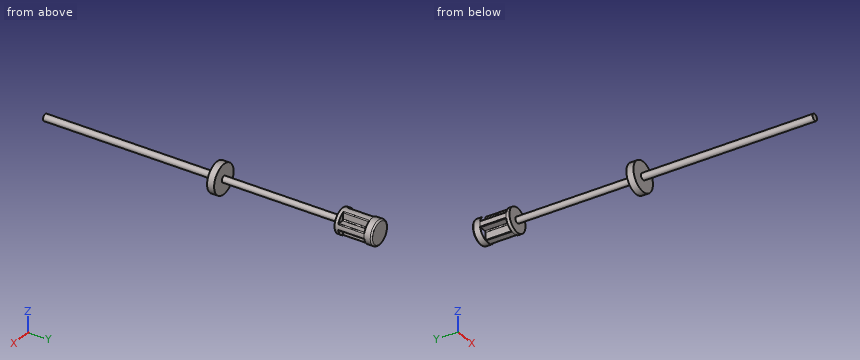
from build123d import *

# Parameters (mm, degrees)
SKETCH1_R           = 0.95
SKETCH5_W           = 4.2
SKETCH5_H           = 2
SKETCH6_R           = 0.885
BOSS_EXTRUDE1_DEPTH = 33.75
SKETCH7_R           = 3.45
BOSS_EXTRUDE2_DEPTH = 1
BOSS_EXTRUDE3_DEPTH = 7.4
SKETCH11_R          = 3.45
BOSS_EXTRUDE4_DEPTH = 2.15
SKETCH12_R          = 5.053108697
SKETCH12_R_2        = 3.449578042
CUT_EXTRUDE1_DEPTH  = 10
FILLET4_R           = 0.4
FILLET5_R           = 0.3
CUT_EXTRUDE2_START  = -3.09
SKETCH15_R          = 0.95
CUT_EXTRUDE2_DEPTH  = 3.09


with BuildPart() as part:
    # Sweep1: sweep along a path in Sketch2
    with BuildLine(Plane(origin=(0, 0, 0), x_dir=(0, 0, -1), z_dir=(1, 0, 0))) as sweep1_path:
        Line((0, 0), (0, 41.9))
        Line((0, 41.9), (0, 51.9))
    # Sketch1 → Sweep1 (sweep)
    with BuildSketch(Plane(origin=(0, 0, 0), x_dir=(1, 0, 0), z_dir=(0, 1, 0))):
        Circle(SKETCH1_R)
    sweep(path=sweep1_path.line)

    # Sketch5 → Revolve1 (revolve)
    with BuildSketch(Plane(origin=(0, 0, 0), x_dir=(0, 0, -1), z_dir=(1, 0, 0))):
        with Locations((-2.1, 52.9)):
            Rectangle(SKETCH5_W, SKETCH5_H)
    revolve(axis=Axis((0, 53.9, 0), (0, -1, 0)))

    # Sketch6 → Boss-Extrude1 (add)
    with BuildSketch(Plane(origin=(0, 53.9, 0), x_dir=(1, 0, 0), z_dir=(0, 1, 0))):
        with Locations(Location((0, 0, 0), (0, 0, 270))):
            Circle(SKETCH6_R)
    extrude(amount=BOSS_EXTRUDE1_DEPTH)

    # Sketch7 → Boss-Extrude2 (add)
    with BuildSketch(Plane(origin=(0, 87.65, 0), x_dir=(1, 0, 0), z_dir=(0, 1, 0))):
        with Locations(Location((0, 0, 0), (0, 0, 270))):
            Circle(SKETCH7_R)
    extrude(amount=BOSS_EXTRUDE2_DEPTH)

    # Sketch8 → Boss-Extrude3 (add)
    with BuildSketch(Plane(origin=(0, 88.65, 0), x_dir=(1, 0, 0), z_dir=(0, 1, 0))):
        Polygon((1.230053166, 0.811701691), (1.230053166, 3.298725541), (-1.010400815, 3.298725541), (-1.010400815, 0.811701691), (-3.353153794, 0.811701691), (-3.353153794, -0.988158581), (-1.010400815, -0.988158581), (-1.010400815, -4.015839789), (1.230053166, -4.015839789), (1.230053166, -0.988158581), (4.082100271, -0.988158581), (4.082100271, 0.811701691), align=None)
    extrude(amount=BOSS_EXTRUDE3_DEPTH)

    # Sketch11 → Boss-Extrude4 (add)
    with BuildSketch(Plane(origin=(0, 96.05, 0), x_dir=(1, 0, 0), z_dir=(0, 1, 0))):
        with Locations(Location((0, 0, 0), (0, 0, 107.029845203))):
            Circle(SKETCH11_R)
    extrude(amount=BOSS_EXTRUDE4_DEPTH)

    # Sketch12 → Cut-Extrude1 (cut)
    with BuildSketch(Plane(origin=(0, 96.05, 0), x_dir=(1, 0, 0), z_dir=(0, 1, 0))):
        Circle(SKETCH12_R)
        with Locations(Location((0, 0, 0), (0, 0, 270))):
            Circle(SKETCH12_R_2, mode=Mode.SUBTRACT)
    extrude(amount=-CUT_EXTRUDE1_DEPTH, mode=Mode.SUBTRACT)

    # Fillet4
    fillet4_edges = [part.edges().sort_by_distance(p)[0] for p in [
        (1.010400815, 98.2, 3.298725541),
    ]]
    fillet(fillet4_edges, radius=FILLET4_R)

    # Fillet5
    # the kernel refuses this fillet: 0.3 mm, written as the material it adds along each edge
    with BuildSketch(Plane(origin=(-1.010400815, 87.9, -0.811701691), x_dir=(-1, 0, 0), z_dir=(0, 1, 0)), Plane(origin=(-1.010400815, 87.9, 0.988158581), x_dir=(0, 0, 1), z_dir=(0, 1, 0)), Plane(origin=(1.230053166, 87.9, -0.811701691), x_dir=(0, 0, -1), z_dir=(0, 1, 0)), Plane(origin=(1.230053166, 87.9, 0.988158581), x_dir=(1, 0, 0), z_dir=(0, 1, 0))) as fillet5_piece_1:
        with BuildLine():
            CenterArc((FILLET5_R, -FILLET5_R), FILLET5_R, 90, 90)
            Line((0, -FILLET5_R), (0, 0))
            Line((0, 0), (FILLET5_R, 0))
        make_face()
    extrude(amount=8.9)
    # the kernel refuses this fillet: 0.3 mm, written as the material it takes off along each edge
    with BuildSketch(Plane(origin=(1.230053166, 88.65, -3.222818313), x_dir=(-0.9453321678939596, 0, -0.32610901911003093), z_dir=(0, 1, 0))) as fillet5_2_piece_1:
        with BuildLine():
            CenterArc((0.213912859, 0.299842347), FILLET5_R, 199.032778114, 72.824800523)
            Line((-0.069686792, 0.202009641), (0, 0))
            ThreePointArc((0, 0), (0.111818707, -0.001812788), (0.223637414, 0))
        make_face()
    extrude(amount=7.4, mode=Mode.SUBTRACT)
    with BuildSketch(Plane(origin=(-1.010400815, 88.65, -3.29828423), x_dir=(0.9657732786653868, 0, -0.2593876909491066), z_dir=(0, 1, 0))) as fillet5_2_piece_2:
        with BuildLine():
            CenterArc((0.230106816, -0.299817566), FILLET5_R, 88.00174108, 76.964525917)
            Line((-0.059625168, -0.222001259), (0, 0))
            ThreePointArc((0, 0), (0.120283777, 0.002097733), (0.240567554, 0))
        make_face()
    extrude(amount=7.4, mode=Mode.SUBTRACT)
    with BuildSketch(Plane(origin=(-3.352719647, 88.65, -0.811701691), x_dir=(-0.1990231654762503, 0, 0.9799947854982765), z_dir=(0, 1, 0))) as fillet5_2_piece_3:
        with BuildLine():
            CenterArc((0.24524038, 0.299792772), FILLET5_R, 191.479842228, 80.649895998)
            Line((-0.048758056, 0.240085822), (0, 0))
            ThreePointArc((0, 0), (0.128194548, -0.002382831), (0.256389095, 0))
        make_face()
    extrude(amount=7.4, mode=Mode.SUBTRACT)
    with BuildSketch(Plane(origin=(-3.30501608, 88.65, 0.988158581), x_dir=(-0.2526309264333675, 0, -0.9675627189022004), z_dir=(0, 1, 0))) as fillet5_2_piece_4:
        with BuildLine():
            CenterArc((0.231775654, -0.29981491), FILLET5_R, 87.987242866, 77.37950549)
            Line((-0.058493162, -0.224025632), (0, 0))
            ThreePointArc((0, 0), (0.121156129, 0.00212828), (0.242312258, 0))
        make_face()
    extrude(amount=7.4, mode=Mode.SUBTRACT)
    with BuildSketch(Plane(origin=(-1.010400815, 88.65, 3.29828423), x_dir=(0.9657732786653864, 0, 0.25938769094910785), z_dir=(0, 1, 0))) as fillet5_2_piece_5:
        with BuildLine():
            CenterArc((0.230106816, 0.299817566), FILLET5_R, 195.033733003, 76.964525917)
            Line((-0.059625168, 0.222001259), (0, 0))
            ThreePointArc((0, 0), (0.120283777, -0.002097733), (0.240567554, 0))
        make_face()
    extrude(amount=7.4, mode=Mode.SUBTRACT)
    with BuildSketch(Plane(origin=(1.230053166, 88.65, 3.222818313), x_dir=(-0.9453321678939602, 0, 0.32610901911002915), z_dir=(0, 1, 0))) as fillet5_2_piece_6:
        with BuildLine():
            CenterArc((0.213912859, -0.299842347), FILLET5_R, 88.142421362, 72.824800523)
            Line((-0.069686792, -0.202009641), (0, 0))
            ThreePointArc((0, 0), (0.111818707, 0.001812788), (0.223637414, 0))
        make_face()
    extrude(amount=7.4, mode=Mode.SUBTRACT)
    with BuildSketch(Plane(origin=(3.30501608, 88.65, 0.988158581), x_dir=(0.2526309264333699, 0, -0.9675627189021997), z_dir=(0, 1, 0))) as fillet5_2_piece_7:
        with BuildLine():
            CenterArc((0.231775654, 0.29981491), FILLET5_R, 194.633251644, 77.37950549)
            Line((-0.058493162, 0.224025632), (0, 0))
            ThreePointArc((0, 0), (0.121156129, -0.00212828), (0.242312258, 0))
        make_face()
    extrude(amount=7.4, mode=Mode.SUBTRACT)
    with BuildSketch(Plane(origin=(3.352719647, 88.65, -0.811701691), x_dir=(0.19902316547625037, 0, 0.9799947854982765), z_dir=(0, 1, 0))) as fillet5_2_piece_8:
        with BuildLine():
            CenterArc((0.24524038, -0.299792772), FILLET5_R, 87.870261774, 80.649895998)
            Line((-0.048758056, -0.240085822), (0, 0))
            ThreePointArc((0, 0), (0.128194548, 0.002382831), (0.256389095, 0))
        make_face()
    extrude(amount=7.4, mode=Mode.SUBTRACT)

    # Sketch15 → Cut-Extrude2 (cut)
    with BuildSketch(Plane.XZ.offset(CUT_EXTRUDE2_START)):
        with Locations(Location((0, 0, 0), (0, 0, 90))):
            Circle(SKETCH15_R)
    extrude(amount=CUT_EXTRUDE2_DEPTH, mode=Mode.SUBTRACT)


solid = part.part
The model under review builds one solid part; all positions refer to its coordinate system, in mm. Give positions to 0.01 mm unless a question says otherwise; leave off trailing zeros. Loops run counter-clockwise (first coordinate to the right, second up) from the corner with the lowest first, then second, coordinate; pieces in that order, holes last. Notation, with made-up numbers: (19.25, -24.5) -> (35.25, -24.5) arc R14 cw to (35.25, -3.5) -> close; hole circle Ø6 at (53.25, 89). An arc over 180 degrees is marked (long way). Write each question's results on one line, items separated by ' | '.
1) Take a section at C-C, the plane y = 44. Give the boundary of the cut face in (x, z).
Conclusion:
outline: circle Ø1.9 at (0, 0)
2) Take a section at B-B, the plane y = 74.5. Give the boundary of the cut face in (x, z) (3 decimals).
Conclusion:
outline: circle Ø1.77 at (0, 0)
3) For line 1 along Y through (x, z) = (2.5, -1.75); line 2 along Y through (x, z) = (3, -1); line 3 along Y through (x, z) = (0.75, -3), list the stretches that pass through material, from the lowest coordinate up. Write a range as from..to.
Conclusion:
line 1: y = 51.9..53.9, 87.65..88.65, 96.05..98.2 | line 2: y = 51.9..53.9, 87.65..88.65, 96.05..98.18 | line 3: y = 51.9..53.9, 87.65..98.2
4) Insertion check: pin 1 Ø1.4 at (x, y) = (-2, 91.5) entering from +Z; pin 2 Ø0.9 at (y, z) = (92, -2.5) entering from +X; pin 3 Ø1.5 at (x, y) = (-1.5, 35.5) entering from +Z; pin 4 Ø1.5 at (y, z) = (34.5, -2.5) entering from -X. Each pin has a flat end and moves straight along its axis. Give the tip position at first contact, or say it passes through.
Conclusion:
pin 1: stops at z = 0.99 | pin 2: stops at x = 1.23 | pin 3: stops at z = 0.58 | pin 4: passes through
